from build123d import *

# Parameters (mm, degrees)
SKETCH1_W           = 200
SKETCH1_H           = 200
BOSS_EXTRUDE1_DEPTH = 10
CUT_EXTRUDE1_REACH  = 143.774
SKETCH2_R           = 6


with BuildPart() as part:
    # Sketch1 → Boss-Extrude1 (new body)
    with BuildSketch(Plane(origin=(0, 0, 0), x_dir=(0, 0, -1), z_dir=(1, 0, 0))):
        Rectangle(SKETCH1_W, SKETCH1_H)
    extrude(amount=BOSS_EXTRUDE1_DEPTH)

    # Sketch2 → Cut-Extrude1 (cut, up to next)
    with BuildSketch(Plane(origin=(10, 0, 0), x_dir=(0, 0, -1), z_dir=(1, 0, 0)), mode=Mode.PRIVATE) as cut_extrude1_sk1:
        with Locations((-55, 40)):
            Circle(SKETCH2_R)
    cut_extrude1_tool1 = extrude(cut_extrude1_sk1.sketch, amount=-CUT_EXTRUDE1_REACH, mode=Mode.PRIVATE) & part.part
    # Sketch2 → Cut-Extrude1 (cut, up to next)
    with BuildSketch(Plane(origin=(10, 0, 0), x_dir=(0, 0, -1), z_dir=(1, 0, 0)), mode=Mode.PRIVATE) as cut_extrude1_sk2:
        with Locations((55, 40)):
            Circle(SKETCH2_R)
    cut_extrude1_tool2 = extrude(cut_extrude1_sk2.sketch, amount=-CUT_EXTRUDE1_REACH, mode=Mode.PRIVATE) & part.part
    add(cut_extrude1_tool1.solids().sort_by_distance((10, 40, 55))[0], mode=Mode.SUBTRACT)
    add(cut_extrude1_tool2.solids().sort_by_distance((10, 40, -55))[0], mode=Mode.SUBTRACT)


solid = part.part
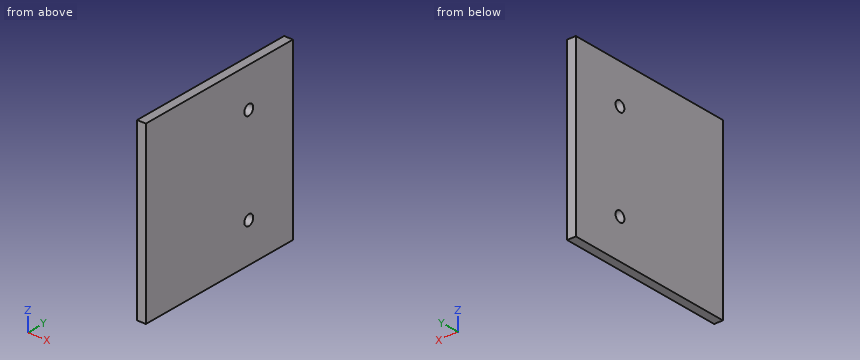
The listing builds one solid part. Answer for the finished solid, in the listing's coordinates (mm). Give positions to 0.01 mm unless a question says otherwise; leave off trailing zeros. Order: outer loops, then holes, each group sorted by start corner. A loop starts at its lowest first (then second) coordinate and runs counter-clockwise, first axis right, second up. Notation, with made-up numbers: (53.25, 78) - (83.25, 78) arc R18 cw to (83.25, 82) - close; hole circle Ø10 at (-36.5, 82). An arc over 180 degrees is marked (long way). One line per item, written item: value. Start each with the question number.
1) A cutting plane is placed at B-B on y = 40. Give the vertices of the cut face in (x, z), then the cut area to 3 significant figures.
2) Find the intervals of material crossed by L1, parallel to Z at x = 2.25, y = 41; L2, parallel to Y at x = 2.5, z = -55; L3, parallel to Y at x = 0.75, z = -60, in increasing order.
3) A cutting plane is placed at A-A on z = 55. Give the vertices of the cut face in (x, y), then the cut area to 3 significant figures.
Answer sheet:
1. outline: (0, -100) - (10, -100) - (10, -61) - (0, -61) - close; (0, -49) - (10, -49) - (10, 49) - (0, 49) - close; (0, 61) - (10, 61) - (10, 100) - (0, 100) - close
1. area: 1,760 mm2
2. L1: z = -100 to -60.92, -49.08 to 49.08, 60.92 to 100
2. L2: y = -100 to 34, 46 to 100
2. L3: y = -100 to 36.68, 43.32 to 100
3. outline: (0, -100) - (10, -100) - (10, 34) - (0, 34) - close; (0, 46) - (10, 46) - (10, 100) - (0, 100) - close
3. area: 1,880 mm2
